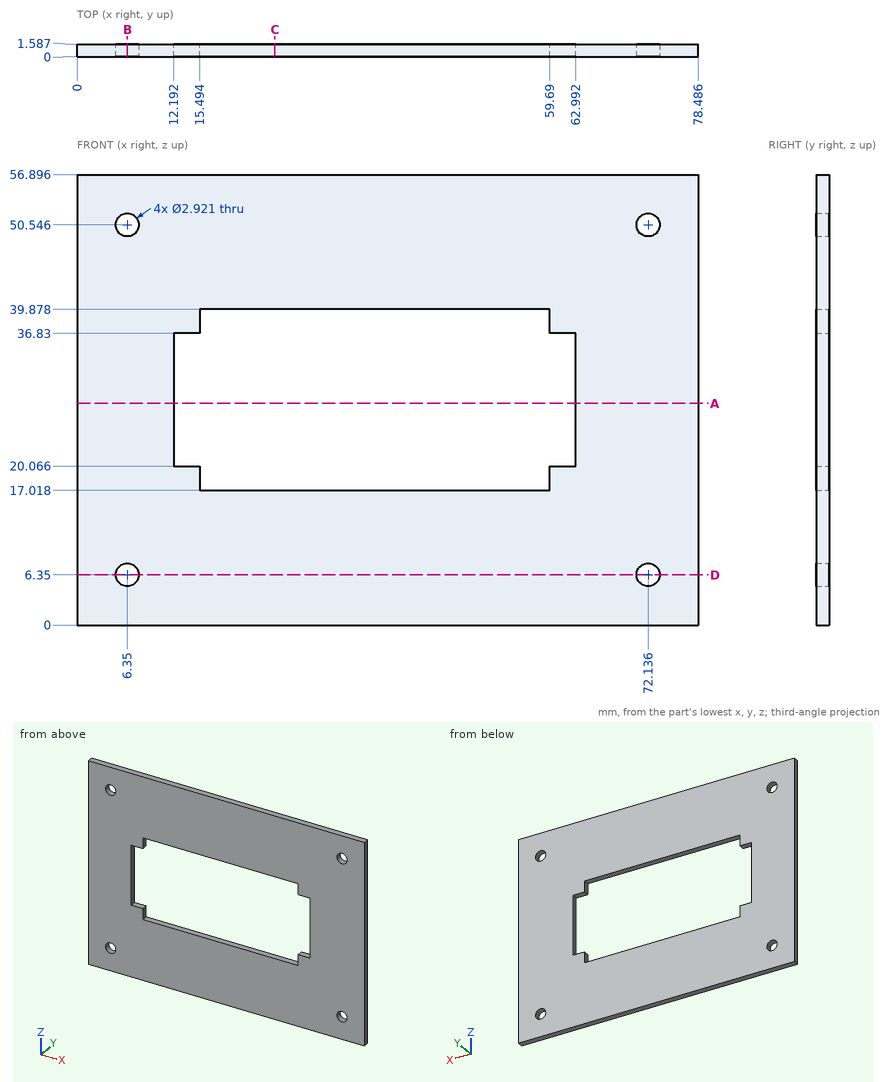
Here's the drawing with two shaded views (mm, measured from the low corner). I have some questions. Give positions to 0.01 mm unless a question says otherwise; leave off trailing zeros. Loops run counter-clockwise (first coordinate to the right, second up) from the corner with the lowest first, then second, coordinate; pieces in that order, holes last. Notation, with made-up numbers: (17, 61) - (43, 61) arc R22 ccw to (43, 84) - close; hole circle Ø5 at (3, 35.25). An arc over 180 degrees is marked (long way). Answer in a Markdown table with one row per item. Add a question column.
Q1. If we section it at A-A (z = 28): List the corners of the cut face in (x, y) for me (1 decimal).
Q2. For pin 1 (4.5 mm diameter, centred on x = 6.35, z = 50.546, fed in from -Y); pin 2 (2.5 mm diameter, centred on x = 72.136, z = 50.546, fed in from +Y), each with a flat end and sliding along its axis, tell me the tip position at first contact or that it passes through.
Q3. Please list where these lines run through material, in increasing order: L1, parallel to Z at x = 6.35, y = 1.15 (1 decimal); L2, parallel to Z at x = 31, y = 0.65 (1 decimal); L3, parallel to X at y = 0.65, z = 35 (1 decimal). Write a range as from..to.
Q4. If we section it at C-C (x = 25): List the corners of the cut face in (y, z) for me (1 decimal).
Q5. If we section it at B-B (x = 6.35): List the corners of the cut face in (y, z) for me (1 decimal).
Q6. If we section it at D-D (z = 6.35): List the corners of the cut face in (x, y) for me (1 decimal), plus the area to 3 significant figures.
The answers:
| question | item | result |
|---|---|---|
| 1 | outline | (0, 0) - (12.2, 0) - (12.2, 1.6) - (0, 1.6) - close; (63, 0) - (78.5, 0) - (78.5, 1.6) - (63, 1.6) - close |
| 2 | pin 1 | stops at y = 0 |
| 2 | pin 2 | passes through |
| 3 | L1 | z = 0..4.9, 7.8..49.1, 52..56.9 |
| 3 | L2 | z = 0..17, 39.9..56.9 |
| 3 | L3 | x = 0..12.2, 63..78.5 |
| 4 | outline | (0, 0) - (1.6, 0) - (1.6, 17) - (0, 17) - close; (0, 39.9) - (1.6, 39.9) - (1.6, 56.9) - (0, 56.9) - close |
| 5 | outline | (0, 0) - (1.6, 0) - (1.6, 4.9) - (0, 4.9) - close; (0, 7.8) - (1.6, 7.8) - (1.6, 49.1) - (0, 49.1) - close; (0, 52) - (1.6, 52) - (1.6, 56.9) - (0, 56.9) - close |
| 6 | outline | (0, 0) - (4.9, 0) - (4.9, 1.6) - (0, 1.6) - close; (7.8, 0) - (70.7, 0) - (70.7, 1.6) - (7.8, 1.6) - close; (73.6, 0) - (78.5, 0) - (78.5, 1.6) - (73.6, 1.6) - close |
| 6 | area | 115 mm^2 |
